Part model, mm, in its own coordinate system. Give positions to 0.01 mm unless a question says otherwise; leave off trailing zeros. Write each loop counter-clockwise with the first axis right and the second up, starting at its lowest first coordinate (ties: lowest second). Pieces come first, ordered by that corner, then holes. Notation, with made-up numbers: (59, -9.75) - (109, -9.75) arc R17 ccw to (109, 8.25) - close; hole circle Ø3 at (-4.75, 14.5). An arc over 180 degrees is marked (long way). Answer as a JSON object with one key per item and string values. Group by question number.
```python
from build123d import *

# Parameters (mm, degrees)
F0_R     = 2.75
F0_R_2   = 3
F1_DEPTH = 5


with BuildPart() as f1:
    # F0 (on Top) → F1 (new body)
    with BuildSketch(Plane.XY):
        with BuildLine():
            Line((-40, 30), (-40, -30))
            Line((-40, -30), (-18.5, -30))
            Line((-18.5, -30), (-18.5, 0))
            ThreePointArc((-18.5, 0), (0, 18.5), (18.5, 0))
            Line((18.5, 0), (18.5, -30))
            Line((18.5, -30), (40, -30))
            Line((40, -30), (40, 30))
            Line((40, 30), (-40, 30))
        make_face()
        with Locations((-21.5, -14.739092)):
            Circle(F0_R, mode=Mode.SUBTRACT)
        with Locations((21.5, -14.739092)):
            Circle(F0_R, mode=Mode.SUBTRACT)
        with Locations((-35, 12)):
            Circle(F0_R_2, mode=Mode.SUBTRACT)
        with Locations((35, 12)):
            Circle(F0_R_2, mode=Mode.SUBTRACT)
        with Locations((0, 22.5)):
            Circle(F0_R, mode=Mode.SUBTRACT)
    extrude(amount=F1_DEPTH)


solid = f1.part
```
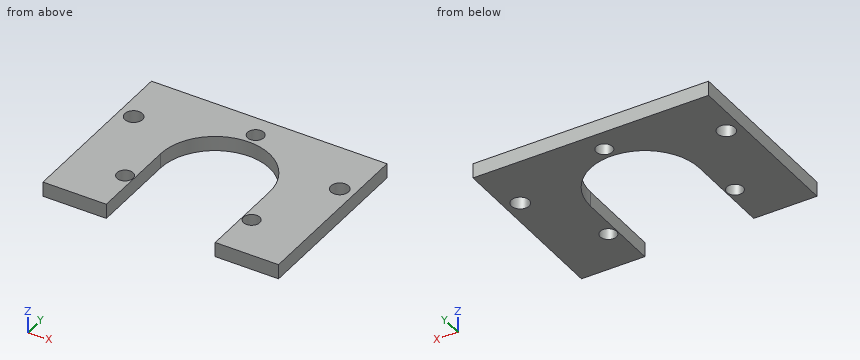
1) Probe line 1 (Y direction, x = -21.5, z = 1.4); line 2 (Y direction, x = 35, z = 2.15); line 3 (X direction, y = -22.5, z = 2.9). List the from-to ranges inside material, lowest first.
2) Band-saw the part on C-C (z = 2.6). List the corners of the cut face in (x, y).
3) Band-saw the part on A-A (y = -5.5). List the corners of the cut face in (x, z).
4) Band-saw the part on B-B (x = 35). List the corners of the cut face in (y, z).
5) Band-saw the part on D-D (x = 13.5). List the corners of the cut face in (y, z), plus the area to 3 significant figures.
Verdict:
{
 "1": {"line 1": "-30 to -17.49, -11.99 to 30", "line 2": "-30 to 9, 15 to 30", "line 3": "-40 to -18.5, 18.5 to 40"},
 "2": {"outline": "(-40, -30) - (-18.5, -30) - (-18.5, 0) arc R18.5 cw to (18.5, 0) - (18.5, -30) - (40, -30) - (40, 30) - (-40, 30) - close; hole circle Ø6 at (-35, 12); hole circle Ø5.5 at (-21.5, -14.74); hole circle Ø5.5 at (0, 22.5); hole circle Ø5.5 at (21.5, -14.74); hole circle Ø6 at (35, 12)"},
 "3": {"outline": "(-40, 0) - (-18.5, 0) - (-18.5, 5) - (-40, 5) - close; (18.5, 0) - (40, 0) - (40, 5) - (18.5, 5) - close"},
 "4": {"outline": "(-30, 0) - (9, 0) - (9, 5) - (-30, 5) - close; (15, 0) - (30, 0) - (30, 5) - (15, 5) - close"},
 "5": {"outline": "(12.65, 0) - (30, 0) - (30, 5) - (12.65, 5) - close", "area": "86.8 mm2"}
}
